Can you work these out from the model? Positions are in its coordinate system, mm. Face numbers are marked on the shaded views. A direction names the side the tool comes from. Give positions to 0.01 mm unless a question says otherwise; leave off trailing zeros. Write each loop counter-clockwise with the first axis right and the second up, starting at its lowest first coordinate (ties: lowest second). Pieces come first, ordered by that corner, then holes.
from build123d import *

# Parameters (mm, degrees)
BOX048_W           = 1.2
BOX048_H           = 6.5
BOX048_DEPTH       = 0.5
BOX049_W           = 1.2
BOX049_H           = 6.5
BOX049_DEPTH       = 0.5
BOX044_W           = 1.2
BOX044_H           = 6.5
BOX044_DEPTH       = 0.5
BOX043_W           = 1.2
BOX043_H           = 6.5
BOX043_DEPTH       = 0.5
BOX039_W           = 1.2
BOX039_H           = 6.5
BOX039_DEPTH       = 0.5
BOX045_W           = 1.2
BOX045_H           = 6.5
BOX045_DEPTH       = 0.5
BOX041_W           = 0.8
BOX041_H           = 6.5
BOX041_DEPTH       = 0.5
BOX040_W           = 0.8
BOX040_H           = 6.5
BOX040_DEPTH       = 0.5
BOX038_W           = 0.8
BOX038_H           = 6.5
BOX038_DEPTH       = 0.5
BOX042_W           = 0.8
BOX042_H           = 6.5
BOX042_DEPTH       = 0.5
BOX047_W           = 0.8
BOX047_H           = 6.5
BOX047_DEPTH       = 0.5
BOX046_W           = 3
BOX046_H           = 8
BOX046_DEPTH       = 4
CYLINDER012_R      = 1.6
CYLINDER012_DEPTH  = 10
CYLINDER011_R      = 1.6
CYLINDER011_DEPTH  = 10
BOX008_W           = 8
BOX008_H           = 20
BOX008_DEPTH       = 4
FILLET002_R        = 1
FILLET_R           = 1
CHAMFER008010_SIZE = 1
CHAMFER008011_SIZE = 0.4


with BuildPart() as cube044:
    # Box048 → Box048 (new body)
    with BuildSketch(Plane(origin=(-4.2, -3.25, 0), x_dir=(1, 0, 0), z_dir=(0, 0, 1))):
        with Locations((0.6, 3.25)):
            Rectangle(BOX048_W, BOX048_H)
    extrude(amount=BOX048_DEPTH)


with BuildPart() as cube045:
    # Box049 → Box049 (new body)
    with BuildSketch(Plane(origin=(-6.2, -3.25, 0), x_dir=(1, 0, 0), z_dir=(0, 0, 1))):
        with Locations((0.6, 3.25)):
            Rectangle(BOX049_W, BOX049_H)
    extrude(amount=BOX049_DEPTH)


with BuildPart() as cube040:
    # Box044 → Box044 (new body)
    with BuildSketch(Plane(origin=(1, -3.25, 0), x_dir=(1, 0, 0), z_dir=(0, 0, 1))):
        with Locations((0.6, 3.25)):
            Rectangle(BOX044_W, BOX044_H)
    extrude(amount=BOX044_DEPTH)


with BuildPart() as cube039:
    # Box043 → Box043 (new body)
    with BuildSketch(Plane(origin=(-1, -3.25, 0), x_dir=(1, 0, 0), z_dir=(0, 0, 1))):
        with Locations((0.6, 3.25)):
            Rectangle(BOX043_W, BOX043_H)
    extrude(amount=BOX043_DEPTH)


with BuildPart() as cube035:
    # Box039 → Box039 (new body)
    with BuildSketch(Plane(origin=(-3, -3.25, 0), x_dir=(1, 0, 0), z_dir=(0, 0, 1))):
        with Locations((0.6, 3.25)):
            Rectangle(BOX039_W, BOX039_H)
    extrude(amount=BOX039_DEPTH)


with BuildPart() as fusion001007011052:
    # Box045 → Box045 (new body)
    with BuildSketch(Plane(origin=(3, -3.25, 0), x_dir=(1, 0, 0), z_dir=(0, 0, 1))):
        with Locations((0.6, 3.25)):
            Rectangle(BOX045_W, BOX045_H)
    extrude(amount=BOX045_DEPTH)

    # Fusion001007011047: union Cube040, Cube039, Cube035
    add(cube040.part)
    add(cube039.part)
    add(cube035.part)


with BuildPart() as fusion001007011052_1:
    # Fusion001007011047 placement: moved
    add(fusion001007011052.part.moved(Location((0.8, 0, 0))))

    # Fusion001007011052: union Cube044, Cube045
    add(cube044.part)
    add(cube045.part)


with BuildPart() as cube037:
    # Box041 → Box041 (new body)
    with BuildSketch(Plane(origin=(2.2, -3.25, -0.5), x_dir=(1, 0, 0), z_dir=(0, 0, 1))):
        with Locations((0.4, 3.25)):
            Rectangle(BOX041_W, BOX041_H)
    extrude(amount=BOX041_DEPTH)


with BuildPart() as cube036:
    # Box040 → Box040 (new body)
    with BuildSketch(Plane(origin=(0.2, -3.25, -0.5), x_dir=(1, 0, 0), z_dir=(0, 0, 1))):
        with Locations((0.4, 3.25)):
            Rectangle(BOX040_W, BOX040_H)
    extrude(amount=BOX040_DEPTH)


with BuildPart() as cube034:
    # Box038 → Box038 (new body)
    with BuildSketch(Plane(origin=(-1.8, -3.25, -0.5), x_dir=(1, 0, 0), z_dir=(0, 0, 1))):
        with Locations((0.4, 3.25)):
            Rectangle(BOX038_W, BOX038_H)
    extrude(amount=BOX038_DEPTH)


with BuildPart() as fusion001007011046:
    # Box042 → Box042 (new body)
    with BuildSketch(Plane(origin=(4.2, -3.25, -0.5), x_dir=(1, 0, 0), z_dir=(0, 0, 1))):
        with Locations((0.4, 3.25)):
            Rectangle(BOX042_W, BOX042_H)
    extrude(amount=BOX042_DEPTH)

    # Fusion001007011046: union Cube037, Cube036, Cube034
    add(cube037.part)
    add(cube036.part)
    add(cube034.part)


with BuildPart() as fusion001007011046_1:
    # Fusion001007011046 placement: moved
    add(fusion001007011046.part.moved(Location((-1.2, 0, 0))))


with BuildPart() as fusion001007011049:
    # Box047 → Box047 (new body)
    with BuildSketch(Plane(origin=(-5, -3.25, -0.5), x_dir=(1, 0, 0), z_dir=(0, 0, 1))):
        with Locations((0.4, 3.25)):
            Rectangle(BOX047_W, BOX047_H)
    extrude(amount=BOX047_DEPTH)

    # Fusion001007011049: union Fusion001007011046
    add(fusion001007011046_1.part)


with BuildPart() as cube042:
    # Box046 → Box046 (new body)
    with BuildSketch(Plane(origin=(-5.5, -4, 0), x_dir=(1, 0, 0), z_dir=(0, 0, 1))):
        with Locations((1.5, 4)):
            Rectangle(BOX046_W, BOX046_H)
    extrude(amount=BOX046_DEPTH)


with BuildPart() as cylinder012:
    # Cylinder012 → Cylinder012 (new body)
    with BuildSketch(Plane(origin=(0, -7, 0), x_dir=(1, 0, 0), z_dir=(0, 0, 1))):
        Circle(CYLINDER012_R)
    extrude(amount=CYLINDER012_DEPTH)


with BuildPart() as fusion017:
    # Cylinder011 → Cylinder011 (new body)
    with BuildSketch(Plane(origin=(0, 7, 0), x_dir=(1, 0, 0), z_dir=(0, 0, 1))):
        Circle(CYLINDER011_R)
    extrude(amount=CYLINDER011_DEPTH)

    # Fusion017: union Cylinder012
    add(cylinder012.part)


with BuildPart() as belt_clamp:
    # Box008 → Box008 (new body)
    with BuildSketch(Plane(origin=(-3, -10, 0), x_dir=(1, 0, 0), z_dir=(0, 0, 1))):
        with Locations((4, 10)):
            Rectangle(BOX008_W, BOX008_H)
    extrude(amount=BOX008_DEPTH)

    # Fillet002
    fillet002_edges = [belt_clamp.edges().sort_by_distance(p)[0] for p in [
        (-3, -10, 2),
        (-3, 10, 2),
        (5, -10, 2),
        (5, 10, 2),
    ]]
    fillet(fillet002_edges, radius=FILLET002_R)

    # Cut008004003012001003001009: cut Fusion017
    add(fusion017.part, mode=Mode.SUBTRACT)

    # Fusion001007011048: union Cube042
    add(cube042.part)

    # Fillet
    fillet_edges = [belt_clamp.edges().sort_by_distance(p)[0] for p in [
        (-5.5, -4, 2),
        (-5.5, 4, 2),
    ]]
    fillet(fillet_edges, radius=FILLET_R)

    # Chamfer008010
    chamfer008010_edges = [belt_clamp.edges().sort_by_distance(p)[0] for p in [
        (-3, 4, 2),
        (-3, -4, 2),
    ]]
    chamfer(chamfer008010_edges, length=CHAMFER008010_SIZE)

    # Fusion001007011051: union Fusion001007011049
    add(fusion001007011049.part)

    # Cut008004003012001003001010001023: cut Fusion001007011052
    add(fusion001007011052_1.part, mode=Mode.SUBTRACT)

    # Chamfer008011
    chamfer008011_edges = [belt_clamp.edges().sort_by_distance(p)[0] for p in [
        (-5.468246, 3.25, 0.25),
        (-5.49203, 3.126004, 0.5),
        (-5.5, 0, 0.5),
        (-5.468246, -3.25, 0.25),
        (-5.49203, -3.126004, 0.5),
    ]]
    chamfer(chamfer008011_edges, length=CHAMFER008011_SIZE)


solid = belt_clamp.part
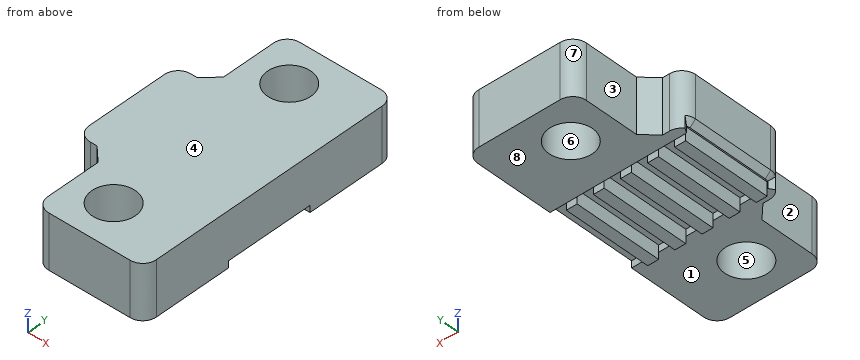
(1) Imagine slicing it at C-C, the plane z = 2.8. Write out the boundary of the cut face in (x, y), plus the area to 3 significant figures.
Returned:
outline: (-5.5, -3) arc R1 ccw to (-4.5, -4) - (-4, -4) - (-3, -5) - (-3, -9) arc R1 ccw to (-2, -10) - (4, -10) arc R1 ccw to (5, -9) - (5, 9) arc R1 ccw to (4, 10) - (-2, 10) arc R1 ccw to (-3, 9) - (-3, 5) - (-4, 4) - (-4.5, 4) arc R1 ccw to (-5.5, 3) - close; hole circle Ø3.2 at (0, -7); hole circle Ø3.2 at (0, 7)
area: 164 mm2
(2) Imagine slicing it at D-D, the plane x = -3.25. Write out the boundary of the cut face in (y, z), plus the area to 4 significant figures.
Returned:
outline: (-4.75, 0) - (-3.25, 0) - (-3.25, 0.5) - (3.25, 0.5) - (3.25, 0) - (4.75, 0) - (4.75, 4) - (-4.75, 4) - close
area: 34.75 mm2
(3) Will these pins go through, and if not, where does the flat tip stop? P1, Ø3, axis at x = -0.5, y = 6.5, coming from the -Z side; P2, Ø0.8, axis at y = -1, z = 0, coming from the +X side; P3, Ø1.2, axis at y = 7.5, z = 1.5, coming from the -X side.
Returned:
P1: stops at z = 0
P2: stops at x = 3.8
P3: stops at x = -3
(4) If we mould it in two halves opening along X, with no side actions, what happens to the marked faces 5, 6, 7 and 8? For each: +X half, -X half, draft (parallel to the pull), parting line (faces both ways), or undercut.
Returned:
face 5: undercut
face 6: undercut
face 7: -X half
face 8: draft
(5) Imagine slicing it at B-B, the plane y = 7. Write out the boundary of the cut face in (x, z), plus the area to 3 significant figures.
Returned:
outline: (-3, 0) - (-1.6, 0) - (-1.6, 4) - (-3, 4) - close; (1.6, 0) - (5, 0) - (5, 4) - (1.6, 4) - close
area: 19.2 mm2
(6) Imagine slicing it at A-A, the plane x = 0. Write out the boundary of the cut face in (y, z), plus the area to 4 significant figures.
Returned:
outline: (-10, 0) - (-8.6, 0) - (-8.6, 4) - (-10, 4) - close; (-5.4, 0) - (-3.25, 0) - (-3.25, 0.5) - (3.25, 0.5) - (3.25, 0) - (5.4, 0) - (5.4, 4) - (-5.4, 4) - close; (8.6, 0) - (10, 0) - (10, 4) - (8.6, 4) - close
area: 51.15 mm2
(7) If I drill on L1, parallel to Y at x = 0, z = 1.1; L2, parallel to Y at x = 1, z = 3.3; L3, parallel to X at y = -7, z = 2.65, over which ranges is the centre line in solid material (lowest first)?
Returned:
L1: y = -10 to -8.6, -5.4 to 5.4, 8.6 to 10
L2: y = -10 to -8.25, -5.75 to 5.75, 8.25 to 10
L3: x = -3 to -1.6, 1.6 to 5
(8) For the marked faces 1, 2, 3 and 4, which set-ups out of +Z, -Z, +X, -X, +Y, -Y let a thin tool reach every point of the face, with its end or its side?
Returned:
face 1: -Z, +X, -X, -Y
face 2: +Z, -Z, -X, -Y
face 3: +Z, -Z, -X, +Y
face 4: +Z, +X, -X, +Y, -Y
